The figure shows three views and two pictorial views of one solid part (mm, origin at its lowest corner). Answer the questions. A direction names the side the tool comes from. Round coordinates to 2 decimals unless told otherwise and drop trailing zeros. Loops run counter-clockwise (first coordinate to the right, second up) from the corner with the lowest first, then second, coordinate; pieces in that order, holes last. Notation, with made-up numbers: (-21.5, 54.25) -> (31.5, 54.25) arc R30 ccw to (31.5, 87.25) -> close; hole circle Ø4 at (5.25, -8.75). An arc over 180 degrees is marked (long way). Use a Markdown table: item, result. Add a question column.
Q1. Section A-A on x = 15.5 is taken. Give the vertices of the cut face in (y, z), then the cut area to 3 significant figures.
Q2. Which of the six approach directions +Z, -Z, +X, -X, +Y, -Y give full straight-line access (tool end or side, diameter ignored) to the marked faces 1 and 2?
Q3. Consider line 1 (Y direction, x = 6, z = 3.25); line 2 (X direction, y = 24.5, z = 3.5). Determine where each line is inside the solid, lowest interval first.
Q4. Section B-B on y = 15.5 is taken. Give the vertices of the cut face in (x, z).
Q5. Section C-C on z = 0.8 is taken. Give the vertices of the cut face in (x, y), then the cut area to 3 significant figures.
Q6. For a pull along Y with two mould halves and no side action, classify the marked faces 3, 4 and 5 as released by +Y, released by -Y, zero draft, split by the parting line, or undercut.
Q7. Given pin 1 Ø5 at (x, y) = (5, 18.5) entering from -Z, flat-ended and moving along its own axis, determine where the tip first touches the part or whether it passes through.
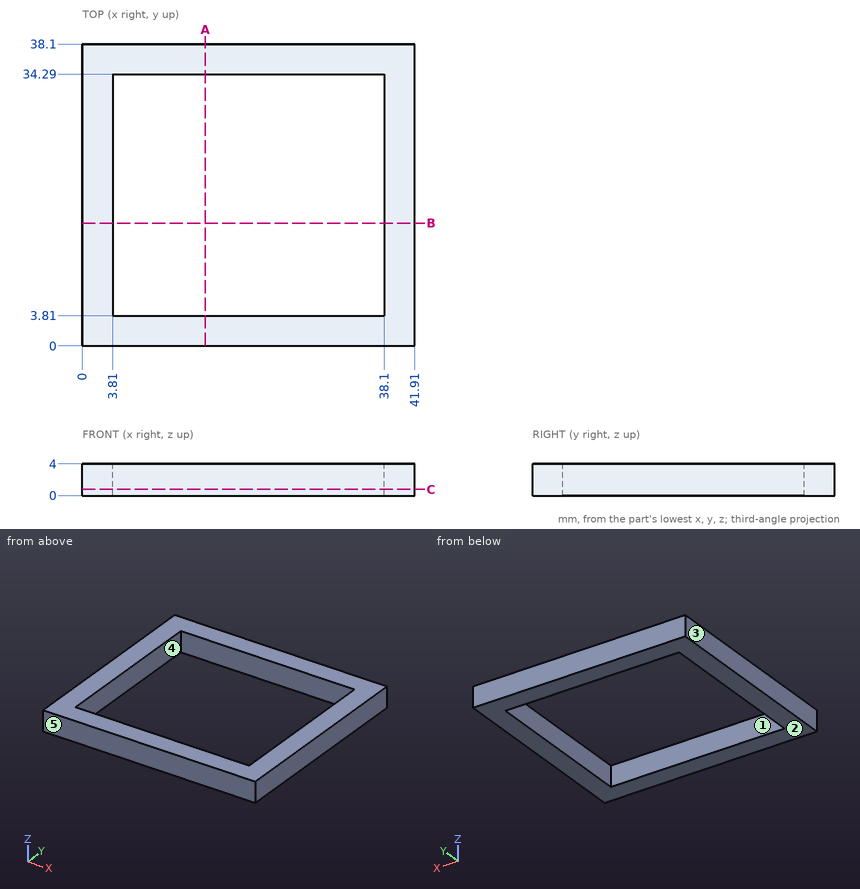
Checked values:
| question | item | result |
|---|---|---|
| 1 | outline | (0, 0) -> (3.81, 0) -> (3.81, 4) -> (0, 4) -> close; (34.29, 0) -> (38.1, 0) -> (38.1, 4) -> (34.29, 4) -> close |
| 1 | area | 30.5 mm2 |
| 2 | face 1 | +Z, -Z |
| 2 | face 2 | -Z, +X, -X, +Y, -Y |
| 3 | line 1 | y = 0 to 3.81, 34.29 to 38.1 |
| 3 | line 2 | x = 0 to 3.81, 38.1 to 41.91 |
| 4 | outline | (0, 0) -> (3.81, 0) -> (3.81, 4) -> (0, 4) -> close; (38.1, 0) -> (41.91, 0) -> (41.91, 4) -> (38.1, 4) -> close |
| 5 | outline | (0, 0) -> (41.91, 0) -> (41.91, 38.1) -> (0, 38.1) -> close; hole (3.81, 3.81) -> (38.1, 3.81) -> (38.1, 34.29) -> (3.81, 34.29) -> close |
| 5 | area | 552 mm2 |
| 6 | face 3 | zero draft |
| 6 | face 4 | undercut |
| 6 | face 5 | released by -Y |
| 7 | pin 1 | stops at z = 0 |
